Can you work these out from the drawing? Everything is in mm from the part's minimum corner. A direction names the side the tool comes from. Coordinates: 2 decimals unless noted, no trailing zeros. Order: outer loops, then holes, each group sorted by start corner. A loop starts at its lowest first (then second) coordinate and runs counter-clockwise, first axis right, second up. Notation, with made-up numbers: (85.5, -9.5) -> (92.5, -9.5) arc R26 ccw to (92.5, 16.5) -> close; hole circle Ø10 at (-19.75, -32.5). An arc over 180 degrees is marked (long way). Put each result on its own line as item: value. Start each with the question number.
Q1. If we section it at B-B (x = 95): Please give me the cut outline in (y, z).
Q2. If we section it at C-C (y = 65): Please give me the cut outline in (x, z), and give its area (3 significant figures).
Q3. For the marked faces 1, 2 and 3, which set-ups out of +Z, -Z, +X, -X, +Y, -Y let a thin tool reach every point of the face, with its end or its side?
Q4. If we section it at A-A (y = 90): Please give me the cut outline in (x, z).
Q5. If we section it at D-D (x = 43.5): Please give me the cut outline in (y, z), and give its area (3 significant figures).
Q6. Will these pins go through, and if not, where does the flat tip stop? pin 1 (6 mm diameter, centred on y = 69.5, z = 5, fed in from -X); pin 2 (9 mm diameter, centred on x = 95, y = 65, fed in from +Z); pin 3 (3.5 mm diameter, centred on x = 95, y = 65, fed in from +Z); pin 4 (1 mm diameter, centred on x = 41, z = 7.5, fed in from +Y).
Q7. Please list where these lines run through material, in increasing order: line 1 along Y through (x, z) = (95, 3.45); line 2 along Y through (x, z) = (10, 6.7); line 3 along X through (y, z) = (14.5, 7).
Q8. We'd pull the mould along X, two halves only. Please class the marked faces 4, 5 and 6: +X half, -X half, draft (parallel to the pull), parting line (faces both ways), or undercut.
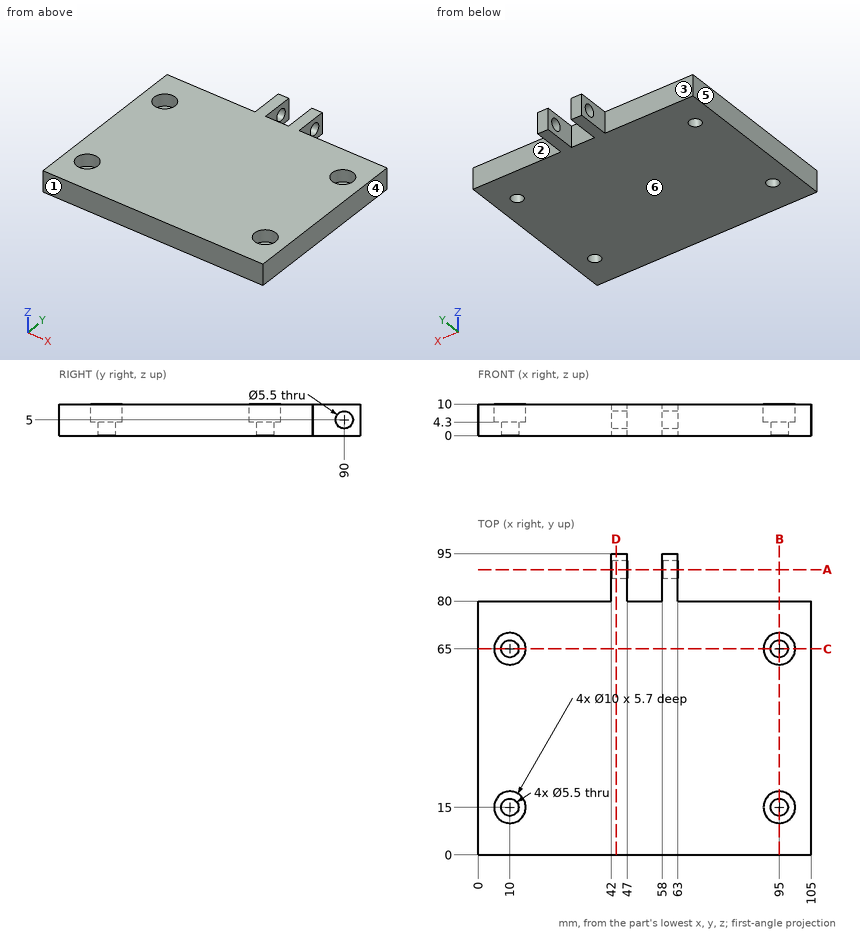
The answers:
1. outline: (0, 0) -> (12.25, 0) -> (12.25, 4.3) -> (10, 4.3) -> (10, 10) -> (0, 10) -> close; (17.75, 0) -> (62.25, 0) -> (62.25, 4.3) -> (60, 4.3) -> (60, 10) -> (20, 10) -> (20, 4.3) -> (17.75, 4.3) -> close; (67.75, 0) -> (80, 0) -> (80, 10) -> (70, 10) -> (70, 4.3) -> (67.75, 4.3) -> close
2. outline: (0, 0) -> (7.25, 0) -> (7.25, 4.3) -> (5, 4.3) -> (5, 10) -> (0, 10) -> close; (12.75, 0) -> (92.25, 0) -> (92.25, 4.3) -> (90, 4.3) -> (90, 10) -> (15, 10) -> (15, 4.3) -> (12.75, 4.3) -> close; (97.75, 0) -> (105, 0) -> (105, 10) -> (100, 10) -> (100, 4.3) -> (97.75, 4.3) -> close
2. area: 889 mm^2
3. face 1: +Z, -Z, +X, -X, -Y
3. face 2: +Z, -Z, +X, +Y
3. face 3: +Z, -Z, -X, +Y
4. outline: (42, 0) -> (47, 0) -> (47, 2.25) -> (42, 2.25) -> close; (42, 7.75) -> (47, 7.75) -> (47, 10) -> (42, 10) -> close; (58, 0) -> (63, 0) -> (63, 2.25) -> (58, 2.25) -> close; (58, 7.75) -> (63, 7.75) -> (63, 10) -> (58, 10) -> close
5. outline: (0, 0) -> (95, 0) -> (95, 10) -> (0, 10) -> close; hole circle Ø5.5 at (90, 5)
5. area: 926 mm^2
6. pin 1: x = 0
6. pin 2: z = 4.3
6. pin 3: through
6. pin 4: y = 80
7. line 1: 0 to 12.25, 17.75 to 62.25, 67.75 to 80
7. line 2: 0 to 10, 20 to 60, 70 to 80
7. line 3: 0 to 5.03, 14.97 to 90.03, 99.97 to 105
8. face 4: +X half
8. face 5: -X half
8. face 6: draft
